Verification items for the finished model (mm, model axes). A direction names the side the tool comes from. Round coordinates to 2 decimals unless told otherwise and drop trailing zeros. Order: outer loops, then holes, each group sorted by start corner. A loop starts at its lowest first (then second) coordinate and runs counter-clockwise, first axis right, second up. Notation, with made-up numbers: (-32.75, 29.5) -> (21.25, 29.5) arc R15 ccw to (21.25, 48.5) -> close; hole circle Ø1 at (59, -18.75). An arc over 180 degrees is marked (long way). Return JSON: item names as keys, results as strings. Group by question number.
Item 1: Sectioned sample at C-C on x = -19.5. Record the cut outline in (y, z).
Item 2: Access from +Z, -Z, +X, -X, +Y, -Y to the whole of each face (thin tool, end or side, straight path). Record for faces 1 (the flat face through (1, 40.132, -1)), 2 (the flat face through (1.8, 37.4, -10.835)), 3 (the flat face through (15, 28, -9.565)).
Item 3: Draft check along Z on faces 4 (the flat face through (15, 28, 8.215)), 5 (the cylindrical face through (14.14, 8.16, -2.96)), 6 (the cylindrical face through (14.14, 8.89, -0.66)), 7 (the flat face through (-5.4, 37.592, -3.1)). Enter one of: pulls with the +Z half, pulls with the -Z half, needs draft (parallel to the pull), parting line crosses it, or undercut.
Item 4: Sectioned sample at D-D on y = 25. Record the cut outline in (x, z).
Item 5: Scan lines: probe 1 along X at (y, z) = (23.5, -4.5); probe 2 along Y at (x, z) = (-31, -8); probe 3 along Y at (x, z) = (2, 6.5). Record each from-to range of solid material in increasing order. Write a range as from..to.
Item 6: Sectioned sample at A-A on x = 13.5. Record the cut outline in (y, z) (3 decimals).
Item 7: Depth check by flat-ended pin: pin 1 Ø1.5 at (y, z) = (37.5, -1.5) entering from -X; pin 2 Ø0.9 at (x, y) = (-36, 28) entering from -Z; pin 3 Ø2 at (x, z) = (-34.09, 4.48) entering from -Y; pin 4 Ø1.4 at (x, z) = (8, 8.5) entering from -Y. Enter the tip coordinate at first touch or a pass-through.
Item 8: Sectioned sample at B-B on z = 7.25. Record the cut outline in (x, y).
```python
from build123d import *

# Parameters (mm, degrees)
SKETCH1_W           = 41.148
SKETCH1_H           = 21.336
BOSS_EXTRUDE1_DEPTH = 37.084
CHAMFER1_SIZE       = 2.54
CHAMFER1_SIZE2      = 14.224
CHAMFER2_SIZE       = 2.54
CHAMFER2_SIZE2      = 4.064
SKETCH3_W           = 18.796
SKETCH3_H           = 20.32
BOSS_EXTRUDE2_DEPTH = 2.54
CHAMFER3_SIZE       = 2.54
CHAMFER3_SIZE_2     = 1.524
SKETCH4_W           = 13.716
SKETCH4_H           = 20.32
BOSS_EXTRUDE3_DEPTH = 3.556
CHAMFER4_SIZE       = 2.54
CHAMFER4_SIZE_2     = 3.048
SKETCH5_R           = 6.858
BOSS_EXTRUDE4_DEPTH = 2.54
BOSS_EXTRUDE4_TAPER = 30
SKETCH6_R           = 3.048
SKETCH6_R_2         = 1.27
BOSS_EXTRUDE5_DEPTH = 4.064
BOSS_EXTRUDE6_DEPTH = 2.032
CHAMFER5_SIZE       = 1.016
CUT_EXTRUDE1_DEPTH  = 1.524
BOSS_EXTRUDE7_DEPTH = 5.08


with BuildPart() as part:
    # Sketch1 → Boss-Extrude1 (new body)
    with BuildSketch(Plane(origin=(0, 0, 0), x_dir=(1, 0, 0), z_dir=(0, 1, 0))):
        with Locations((-8.942205534, 0.674656126)):
            Rectangle(SKETCH1_W, SKETCH1_H)
    extrude(amount=BOSS_EXTRUDE1_DEPTH)

    # Chamfer1
    chamfer1_edges = [part.edges().sort_by_distance(p)[0] for p in [
        (-29.516205534, 37.084, -0.674656126),
    ]]
    chamfer1_side = [part.faces().sort_by_distance(p)[0] for p in [
        (-29.516205534, 18.542, -0.674656126),
    ]]
    chamfer(chamfer1_edges, length=CHAMFER1_SIZE, length2=CHAMFER1_SIZE2, reference=chamfer1_side[0])

    # Chamfer2
    chamfer2_edges = [part.edges().sort_by_distance(p)[0] for p in [
        (11.631794466, 37.084, -0.674656126),
    ]]
    chamfer2_side = [part.faces().sort_by_distance(p)[0] for p in [
        (11.631794466, 18.542, -0.674656126),
    ]]
    chamfer(chamfer2_edges, length=CHAMFER2_SIZE, length2=CHAMFER2_SIZE2, reference=chamfer2_side[0])

    # Sketch3 → Boss-Extrude2 (add)
    with BuildSketch(Plane(origin=(0, 35.052, 0), x_dir=(1, 0, 0), z_dir=(0, 1, 0))):
        with Locations((1.217794466, 0.674656126)):
            Rectangle(SKETCH3_W, SKETCH3_H)
    extrude(amount=BOSS_EXTRUDE2_DEPTH)

    # Chamfer3
    # the kernel refuses this chamfer: 2.54, 1.524 mm, written as the material it takes off along each edge
    with BuildSketch(Plane(origin=(10.615794466, 37.592, -17.403759313), x_dir=(0.019893418958582338, -0.9998021063601228, 0), z_dir=(0, 0, 1))) as chamfer3_piece_1_section:
        Polygon((CHAMFER3_SIZE * 0.99980210636, -CHAMFER3_SIZE * 0.0198934189586), (-CHAMFER3_SIZE_2 * 0.0198934189586, -CHAMFER3_SIZE_2 * 0.99980210636), (0, 0), align=None)
    chamfer3_piece_1 = extrude(amount=33.458206374, mode=Mode.PRIVATE)
    chamfer3_piece_1 = split(chamfer3_piece_1, bisect_by=Plane(origin=(9.549275809, 35.845574161, -0.674656126), z_dir=(0.5299989400031799, 0.8479983040050881, 0)), keep=Keep.TOP, mode=Mode.PRIVATE)
    add(chamfer3_piece_1, mode=Mode.SUBTRACT)

    # Sketch4 → Boss-Extrude3 (add)
    with BuildSketch(Plane(origin=(0, 34.544, 0), x_dir=(1, 0, 0), z_dir=(0, 1, 0))):
        with Locations((-16.562205534, 0.674656126)):
            Rectangle(SKETCH4_W, SKETCH4_H)
    extrude(amount=BOSS_EXTRUDE3_DEPTH)

    # Chamfer4
    # the kernel refuses this chamfer: 3.048, 2.54 mm, written as the material it takes off along each edge
    with BuildSketch(Plane(origin=(-23.420205534, 38.1, 17.341921223), x_dir=(-0.03575241599375306, -0.9993606780090006, 0), z_dir=(0, 0, -1))) as chamfer4_piece_1_section:
        Polygon((CHAMFER4_SIZE * 0.999360678009, -CHAMFER4_SIZE * 0.0357524159938), (-CHAMFER4_SIZE_2 * 0.0357524159938, -CHAMFER4_SIZE_2 * 0.999360678009), (0, 0), align=None)
    chamfer4_piece_1 = extrude(amount=36.0331547, mode=Mode.PRIVATE)
    chamfer4_piece_1 = split(chamfer4_piece_1, bisect_by=Plane(origin=(-22.151753268, 35.859080762, -0.674656126), z_dir=(-0.17579063848365747, 0.984427575508482, 0)), keep=Keep.TOP, mode=Mode.PRIVATE)
    add(chamfer4_piece_1, mode=Mode.SUBTRACT)

    # Sketch5 → Boss-Extrude4 (add)
    with BuildSketch(Plane(origin=(0, 37.592, 0), x_dir=(1, 0, 0), z_dir=(0, 1, 0))):
        with Locations((1.471794466, 0.674656126)):
            Circle(SKETCH5_R)
    extrude(amount=BOSS_EXTRUDE4_DEPTH, taper=BOSS_EXTRUDE4_TAPER)

    # Sketch6 → Boss-Extrude5 (add)
    with BuildSketch(Plane(origin=(0, 40.132, 0), x_dir=(1, 0, 0), z_dir=(0, 1, 0))):
        with Locations(Location((1.471794466, 0.674656126, 0), (0, 0, 270))):
            Circle(SKETCH6_R)
        with Locations(Location((1.471794466, 0.674656126, 0), (0, 0, 270))):
            Circle(SKETCH6_R_2, mode=Mode.SUBTRACT)
    extrude(amount=BOSS_EXTRUDE5_DEPTH)

    # Sketch7 → Boss-Extrude6 (add)
    with BuildSketch(Plane(origin=(0, 27.432, 0), x_dir=(-1, 0, 0), z_dir=(0, -1, 0))):
        with BuildLine():
            Line((29.516205534, 9.564656126), (36.628205534, 9.564656126))
            Line((36.628205534, 9.564656126), (36.628205534, 6.84497112))
            Line((36.628205534, 6.84497112), (35.547324446, 6.84497112))
            ThreePointArc((35.547324446, 6.84497112), (32.310205534, 5.82897112), (35.547324446, 4.81297112))
            Line((35.547324446, 4.81297112), (36.628205534, 4.81297112))
            Line((36.628205534, 4.81297112), (36.628205534, -3.463658867))
            Line((36.628205534, -3.463658867), (35.547324446, -3.463658867))
            ThreePointArc((35.547324446, -3.463658867), (32.310205534, -4.479658867), (35.547324446, -5.495658867))
            Line((35.547324446, -5.495658867), (36.628205534, -5.495658867))
            Line((36.628205534, -5.495658867), (36.628205534, -8.215343874))
            Line((36.628205534, -8.215343874), (29.516205534, -8.215343874))
            Line((29.516205534, -8.215343874), (29.516205534, 9.564656126))
        make_face()
    boss_extrude6 = extrude(amount=-BOSS_EXTRUDE6_DEPTH)

    # Mirror1: Boss-Extrude6 across plane
    add(boss_extrude6.mirror(Plane(origin=(-8.942205534, 0, 0), x_dir=(0, 0, 1), z_dir=(1, 0, 0))))

    # Chamfer5
    chamfer5_edges = [part.edges().sort_by_distance(p)[0] for p in [
        (-8.942205534, 0, -11.342656126),
        (11.631794466, 0, -0.674656126),
        (-8.942205534, 0, 9.993343874),
        (-29.516205534, 0, -0.674656126),
    ]]
    chamfer(chamfer5_edges, length=CHAMFER5_SIZE)

    # Sketch8 → Cut-Extrude1 (cut)
    with BuildSketch(Plane.XZ):
        with BuildLine():
            Line((-29.516205534, 9.993343874), (-24.944205534, 9.993343874))
            Line((-24.944205534, 9.993343874), (-24.944205534, 9.485343874))
            ThreePointArc((-24.944205534, 9.485343874), (-26.134523575, 6.611661915), (-29.008205534, 5.421343874))
            Line((-29.008205534, 5.421343874), (-29.516205534, 5.421343874))
            Line((-29.516205534, 5.421343874), (-29.516205534, 9.993343874))
        make_face()
        with BuildLine():
            Line((-29.516205534, -11.342656126), (-29.516205534, -6.770656126))
            Line((-29.516205534, -6.770656126), (-29.008205534, -6.770656126))
            ThreePointArc((-29.008205534, -6.770656126), (-26.134523575, -7.960974168), (-24.944205534, -10.834656126))
            Line((-24.944205534, -10.834656126), (-24.944205534, -11.342656126))
            Line((-24.944205534, -11.342656126), (-29.516205534, -11.342656126))
        make_face()
        with BuildLine():
            Line((11.631794466, -11.342656126), (7.059794466, -11.342656126))
            Line((7.059794466, -11.342656126), (7.059794466, -10.834656126))
            ThreePointArc((7.059794466, -10.834656126), (8.250112508, -7.960974168), (11.123794466, -6.770656126))
            Line((11.123794466, -6.770656126), (11.631794466, -6.770656126))
            Line((11.631794466, -6.770656126), (11.631794466, -11.342656126))
        make_face()
        with BuildLine():
            Line((11.631794466, 9.993343874), (11.631794466, 5.421343874))
            Line((11.631794466, 5.421343874), (11.123794466, 5.421343874))
            ThreePointArc((11.123794466, 5.421343874), (8.250112508, 6.611661915), (7.059794466, 9.485343874))
            Line((7.059794466, 9.485343874), (7.059794466, 9.993343874))
            Line((7.059794466, 9.993343874), (11.631794466, 9.993343874))
        make_face()
    extrude(amount=-CUT_EXTRUDE1_DEPTH, mode=Mode.SUBTRACT)

    # Sketch9 → Boss-Extrude7 (add)
    with BuildSketch(Plane(origin=(11.631794466, 0, 0), x_dir=(0, 0, -1), z_dir=(1, 0, 0))):
        with BuildLine():
            Line((-0.098001741, 8.255), (-0.076686006, 8.255))
            ThreePointArc((-0.076686006, 8.255), (0.674656126, 8.89), (1.425998259, 8.255))
            Line((1.425998259, 8.255), (1.447313994, 8.255))
            ThreePointArc((1.447313994, 8.255), (2.960656126, 8.128), (1.447313994, 8.001))
            Line((1.447313994, 8.001), (1.425998259, 8.001))
            ThreePointArc((1.425998259, 8.001), (0.674656126, 7.366), (-0.076686006, 8.001))
            Line((-0.076686006, 8.001), (-0.098001741, 8.001))
            ThreePointArc((-0.098001741, 8.001), (-1.611343874, 8.128), (-0.098001741, 8.255))
        make_face()
    extrude(amount=BOSS_EXTRUDE7_DEPTH)


solid = part.part
```
Recorded:
{
 "1": {"outline": "(0, -10.33) -> (1.02, -11.34) -> (36.33, -11.34) -> (36.33, -10.83) -> (38.1, -10.83) -> (38.1, 9.49) -> (36.33, 9.49) -> (36.33, 9.99) -> (1.02, 9.99) -> (0, 8.98) -> close"},
 "2": {"face 1": "+Y", "face 2": "-Z, +X, +Y", "face 3": "-Z, +X, +Y, -Y"},
 "3": {"face 4": "pulls with the +Z half", "face 5": "undercut", "face 6": "undercut", "face 7": "needs draft"},
 "4": {"outline": "(-29.52, -11.34) -> (11.63, -11.34) -> (11.63, 9.99) -> (-29.52, 9.99) -> close"},
 "5": {"probe 1": "-29.52..11.63", "probe 2": "27.43..29.46", "probe 3": "0..37.59"},
 "6": {"outline": "(8.001, -1.447) arc R0.762 ccw (long way) to (8.255, -1.447) -> (8.255, -1.426) arc R0.762 ccw to (8.255, 0.077) -> (8.255, 0.098) arc R0.762 ccw (long way) to (8.001, 0.098) -> (8.001, 0.077) arc R0.762 ccw to (8.001, -1.426) -> close; (27.432, -9.565) -> (29.464, -9.565) -> (29.464, 8.215) -> (27.432, 8.215) -> close"},
 "7": {"pin 1": "x = -21.99", "pin 2": "z = -9.56", "pin 3": "through", "pin 4": "y = 1.52"},
 "8": {"outline": "(-36.63, 27.43) -> (-29.52, 27.43) -> (-29.52, 1.52) -> (-25.61, 1.52) -> (-25.61, 0) -> (7.73, 0) -> (7.73, 1.52) -> (11.63, 1.52) -> (11.63, 27.43) -> (18.74, 27.43) -> (18.74, 29.46) -> (11.63, 29.46) -> (11.63, 34.54) -> (10.49, 35.26) -> (9.09, 37.59) -> (-8.18, 37.59) -> (-8.18, 37.08) -> (-9.7, 37.08) -> (-9.7, 38.1) -> (-20.37, 38.1) -> (-23.31, 35.65) -> (-29.52, 34.54) -> (-29.52, 29.46) -> (-36.63, 29.46) -> close"}
}
